Here's how the part is built. I have some questions about the finished solid (model axes, mm). A direction names the side the tool comes from. Coordinates: 2 decimals unless noted, no trailing zeros. Write each loop counter-clockwise with the first axis right and the second up, starting at its lowest first coordinate (ties: lowest second). Pieces come first, ordered by that corner, then holes. Notation, with made-up numbers: (73.25, -11) - (105.25, -11) arc R34 ccw to (105.25, 27) - close; hole circle Ø2 at (9.5, 87.25). An arc over 180 degrees is marked (long way). Answer in a Markdown table with one row per item. Add a question column.
Item 1: Imagine slicing it at D-D (x = 28.5). Please give me the cut outline in (y, z).
Item 2: I'm going to push flat-ended pins straight in: pin 1 (4 mm diameter, centred on x = -21.5, z = 373, fed in from -Y); pin 2 (6.5 mm diameter, centred on x = -40, y = -30, fed in from +Z); pin 3 (8 mm diameter, centred on x = 20.5, z = 158.5, fed in from +Y); pin 4 (13 mm diameter, centred on x = 40, y = -30, fed in from -Z). Where does each tip first touch, or does it pass through?
Item 3: Imagine slicing it at B-B (y = 7). Please give me the cut outline in (x, z), plus the area to 3 significant figures.
Item 4: Imagine slicing it at C-C (x = -5.5). Please give me the cut outline in (y, z), plus the area to 3 significant figures.
Item 5: Which directions (+Z, -Z, +X, -X, +Y, -Y) give clear straight access to the entire face, cutting with the end or side of a thin tool? Please do faces 1 (the face through (0, -20, 345)), 2 (the face through (0, -18.5, 345)), 3 (the face through (-20, 0, 345)).
Item 6: We'd pull the mould along X, two halves only. Please class faces 4 (the face through (0, 18.5, 345)), 5 (the face through (20, 0, 345)), 6 (the face through (-2, -19, 0)): +X half, -X half, draft (parallel to the pull), parting line (faces both ways), or undercut.
Item 7: If I drill on probe 1 along Y at (x, z) = (-40, 706.25); probe 2 along X at (y, z) = (12.5, 286.5), over which ranges is the centre line in solid material (lowest first)? Write a range as from..to.
Item 8: Imagine slicing it at A-A (z = 151). Please give me the cut outline in (x, y), plus the area to 3 significant figures.
from build123d import *

# Parameters (mm, degrees)
ESQUISSE1_W             = 40
ESQUISSE1_H             = 40
ESQUISSE1_W_2           = 37
ESQUISSE1_H_2           = 37
BOSS_EXTRU_1_DEPTH      = 700
BOSS_EXTRU_2_DEPTH      = 10
ESQUISSE3_R             = 4
ENL_V_MAT_EXTRU_1_DEPTH = 10


with BuildPart() as part:
    # Esquisse1 → Boss.-Extru.1 (new body)
    with BuildSketch(Plane.XY):
        Rectangle(ESQUISSE1_W, ESQUISSE1_H)
        Rectangle(ESQUISSE1_W_2, ESQUISSE1_H_2, mode=Mode.SUBTRACT)
    extrude(amount=BOSS_EXTRU_1_DEPTH)

    # Esquisse2 → Boss.-Extru.2 (add)
    with BuildSketch(Plane.XY.offset(700)):
        with BuildLine():
            Line((-40, -40), (40, -40))
            ThreePointArc((40, -40), (47.071067812, -37.071067812), (50, -30))
            Line((50, -30), (50, 30))
            ThreePointArc((50, 30), (47.071067812, 37.071067812), (40, 40))
            Line((40, 40), (-40, 40))
            ThreePointArc((-40, 40), (-47.071067812, 37.071067812), (-50, 30))
            Line((-50, 30), (-50, -30))
            ThreePointArc((-50, -30), (-47.071067812, -37.071067812), (-40, -40))
        make_face()
    extrude(amount=BOSS_EXTRU_2_DEPTH)

    # Esquisse3 → Enlèv. mat.-Extru.1 (cut)
    with BuildSketch(Plane(origin=(0, 0, 700), x_dir=(-1, 0, 0), z_dir=(0, 0, -1))):
        with Locations((40, 30)):
            Circle(ESQUISSE3_R)
        with Locations((-40, 30)):
            Circle(ESQUISSE3_R)
        with Locations((-40, -30)):
            Circle(ESQUISSE3_R)
        with Locations((40, -30)):
            Circle(ESQUISSE3_R)
    extrude(amount=-ENL_V_MAT_EXTRU_1_DEPTH, mode=Mode.SUBTRACT)


solid = part.part
Here are the results:
| question | item | result |
|---|---|---|
| 1 | outline | (-40, 700) - (40, 700) - (40, 710) - (-40, 710) - close |
| 2 | pin 1 | stops at y = -20 |
| 2 | pin 2 | passes through |
| 2 | pin 3 | stops at y = 20 |
| 2 | pin 4 | stops at z = 700 |
| 3 | outline | (-50, 700) - (-20, 700) - (-20, 0) - (-18.5, 0) - (-18.5, 700) - (18.5, 700) - (18.5, 0) - (20, 0) - (20, 700) - (50, 700) - (50, 710) - (-50, 710) - close |
| 3 | area | 3,100 mm2 |
| 4 | outline | (-40, 700) - (-20, 700) - (-20, 0) - (-18.5, 0) - (-18.5, 700) - (18.5, 700) - (18.5, 0) - (20, 0) - (20, 700) - (40, 700) - (40, 710) - (-40, 710) - close |
| 4 | area | 2,900 mm2 |
| 5 | face 1 | -Z, +X, -X, -Y |
| 5 | face 2 | -Z |
| 5 | face 3 | -Z, -X, +Y, -Y |
| 6 | face 4 | undercut |
| 6 | face 5 | +X half |
| 6 | face 6 | draft |
| 7 | probe 1 | y = -40..-34, -26..26, 34..40 |
| 7 | probe 2 | x = -20..-18.5, 18.5..20 |
| 8 | outline | (-20, -20) - (20, -20) - (20, 20) - (-20, 20) - close; hole (-18.5, -18.5) - (18.5, -18.5) - (18.5, 18.5) - (-18.5, 18.5) - close |
| 8 | area | 231 mm2 |
